from build123d import *

# Parameters (mm, degrees)
F0_R     = 16
F1_DEPTH = 5
F2_DEPTH = 3
F3_R     = 9
F4_DEPTH = 5.001


with BuildPart() as f1:
    # F0 (on Top) → F1 (new body)
    with BuildSketch(Plane.XY):
        with BuildLine():
            ThreePointArc((20.850659, -2.5), (20.962632, -1.252228), (21, 0))
            ThreePointArc((21, 0), (20.962632, 1.252228), (20.850659, 2.5))
            ThreePointArc((20.850659, 2.5), (-21, 0), (20.850659, -2.5))
        make_face()
        Circle(F0_R, mode=Mode.SUBTRACT)
        with BuildLine():
            ThreePointArc((20.850659, 2.5), (20.962632, 1.252228), (21, 0))
            ThreePointArc((21, 0), (20.962632, -1.252228), (20.850659, -2.5))
            Line((20.850659, -2.5), (56, -2.5))
            Line((56, -2.5), (56, 0))
            Line((56, 0), (56, 2.5))
            Line((56, 2.5), (20.850659, 2.5))
        make_face()
        Circle(F0_R)
    extrude(amount=F1_DEPTH)

    # F0 (on Top) → F2 (cut)
    with BuildSketch(Plane.XY):
        Circle(F0_R)
    extrude(amount=F2_DEPTH, mode=Mode.SUBTRACT)

    # F3 (on face) → F4 (cut, through all)
    with BuildSketch(Plane.XY.offset(5)):
        Circle(F3_R)
    extrude(amount=-F4_DEPTH, mode=Mode.SUBTRACT)


solid = f1.part
Build history of the part. All positions in model axes, mm. A direction names the side the tool comes from. Round coordinates to 2 decimals unless told otherwise and drop trailing zeros. Loops run counter-clockwise (first coordinate to the right, second up) from the corner with the lowest first, then second, coordinate; pieces in that order, holes last. Notation, with made-up numbers: (26, 60) -> (44, 60) arc R16 cw to (44, 69) -> close; hole circle Ø1 at (32, 85.25). An arc over 180 degrees is marked (long way). Answer in a Markdown table with one row per item.
Item 1: Pin check, flat tips, straight feed: pin 1 (9.5 mm diameter, centred on x = -7, y = -5.5, fed in from -Z); pin 2 (1.5 mm diameter, centred on x = 36.5, z = 3, fed in from -Y); pin 3 (1.5 mm diameter, centred on y = -6.5, z = 2.5, fed in from +X). Stop position of each tip, or through.
Answers below:
| item | result |
|---|---|
| pin 1 | stops at z = 3 |
| pin 2 | stops at y = -2.5 |
| pin 3 | stops at x = 20.2 |
Item 2: Saw through at A-A (y = 0). Write the cut outline in (x, z), and give its area (3 significant figures).
Answers below:
| item | result |
|---|---|
| outline | (-21, 0) -> (-16, 0) -> (-16, 3) -> (-9, 3) -> (-9, 5) -> (-21, 5) -> close; (9, 3) -> (16, 3) -> (16, 0) -> (56, 0) -> (56, 5) -> (9, 5) -> close |
| area | 253 mm² |
Item 3: Saw through at C-C (z = 1.5). Write the cut outline in (x, y).
Answers below:
| item | result |
|---|---|
| outline | (20.85, -2.5) -> (56, -2.5) -> (56, 2.5) -> (20.85, 2.5) arc R21 ccw (long way) to start; hole circle Ø32 at (0, 0) |
Item 4: Saw through at D-D (x = 26). Write the cut outline in (y, z), and give its area (3 significant figures).
Answers below:
| item | result |
|---|---|
| outline | (-2.5, 0) -> (2.5, 0) -> (2.5, 5) -> (-2.5, 5) -> close |
| area | 25.0 mm² |
Item 5: Drill centre lines: L1, parallel to Y at x = 0, z = 0.6; L2, parallel to Y at x = 0, z = 3.6; L3, parallel to Z at x = -4.5, y = -9.5. Where is each one in solid material? Low to high. Write a range as [from, to].
Answers below:
| item | result |
|---|---|
| L1 | y = [-21, -16], [16, 21] |
| L2 | y = [-21, -9], [9, 21] |
| L3 | z = [3, 5] |
Item 6: Saw through at B-B (x = 0). Write the cut outline in (y, z), and give its area (3 significant figures).
Answers below:
| item | result |
|---|---|
| outline | (-21, 0) -> (-16, 0) -> (-16, 3) -> (-9, 3) -> (-9, 5) -> (-21, 5) -> close; (9, 3) -> (16, 3) -> (16, 0) -> (21, 0) -> (21, 5) -> (9, 5) -> close |
| area | 78.0 mm² |
Item 7: Mould opens along X. For faces 1 (the cylindrical face through (-20.98, 0.89, 2.46)), 2 (the cylindrical face through (-1.172, 8.923, 4.014)), 3 (the flat face through (17, -1, 0)) say: +X half, -X half, draft (parallel to the pull), parting line (faces both ways), or undercut.
Answers below:
| item | result |
|---|---|
| face 1 | parting line |
| face 2 | undercut |
| face 3 | draft |
Item 8: Which spindle directions (+Z, -Z, +X, -X, +Y, -Y) get a long thin tool onto all of the face, cutting with end or side? Do faces 4 (the flat face through (56, 0, 2)), 5 (the flat face through (8, 5, 5)), 6 (the flat face through (7, -7, 3)), 7 (the flat face through (38, -2.5, 2)), 8 (the flat face through (39, 2.5, 2)). Say none if no direction does.
Answers below:
| item | result |
|---|---|
| face 4 | +Z, -Z, +X, +Y, -Y |
| face 5 | +Z, +X, -X, +Y, -Y |
| face 6 | -Z |
| face 7 | +Z, -Z, +X, -Y |
| face 8 | +Z, -Z, +X, +Y |
